Could you check a few things on this drawing? It's one solid part, dimensions in mm from its lowest x, y, z. A direction names the side the tool comes from. Give positions to 0.01 mm unless a question says otherwise; leave off trailing zeros. Order: outer loops, then holes, each group sorted by start corner. A loop starts at its lowest first (then second) coordinate and runs counter-clockwise, first axis right, second up. Notation, with made-up numbers: (73.5, 26) -> (79.5, 26) arc R15 ccw to (79.5, 46) -> close; hole circle Ø6 at (-31, -1). An arc over 180 degrees is marked (long way). Use one line per item in the form item = value. Start each with the question number.
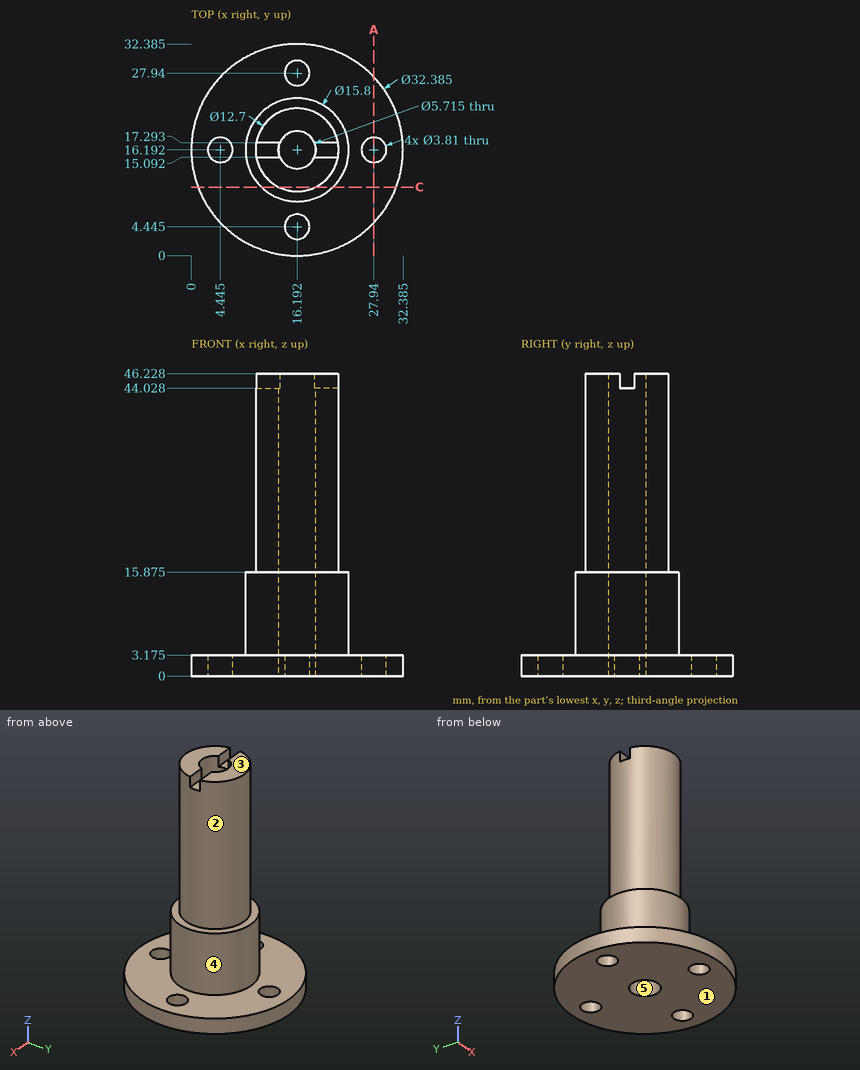
(1) Imagine slicing it at A-A (x = 27.94). Write out the boundary of the cut face in (y, z) (1 decimal).
(2) Please list where these lines run through material, in increasing order: probe 1 along Y at (x, z) = (16, 43.5) (1 decimal); probe 2 along Z at (x, y) = (18, 2) (1 decimal); probe 3 along X at (y, z) = (18, 25.5) (1 decimal).
(3) We'd pull the mould along X, two halves only. Please class the marked faces 3, 4 and 5: pulls with the +X half, pulls with the -X half, needs draft (parallel to the pull), parting line crosses it, or undercut.
(4) I'm going to push flat-ended pins straight in: pin 1 Ø6 at (y, z) = (7.5, 8) entering from -X (1 decimal); pin 2 Ø1.1 at (x, z) = (12, 45) entering from -Y; pin 3 Ø0.7 at (x, z) = (21.5, 44.5) entering from -Y (1 decimal). Where does each tip first touch, or does it pass through?
(5) Which directions (+Z, -Z, +X, -X, +Y, -Y) give clear straight access to the entire face, cutting with the end or side of a thin tool? Please do the marked faces 1 and 2.
(6) Imagine slicing it at C-C (y = 10.5). Write out the boundary of the cut face in (x, z) (1 decimal).
Calculated:
q1.outline = (5, 0) -> (14.3, 0) -> (14.3, 3.2) -> (5, 3.2) -> close; (18.1, 0) -> (27.3, 0) -> (27.3, 3.2) -> (18.1, 3.2) -> close
q2.probe_1 = 9.8 to 13.3, 19 to 22.5
q2.probe_2 = 0 to 3.2
q2.probe_3 = 10.1 to 14, 18.4 to 22.3
q3.face_3 = needs draft
q3.face_4 = parting line crosses it
q3.face_5 = undercut
q4.pin_1 = 10.7
q4.pin_2 = 10.99
q4.pin_3 = 12.2
q5.face_1 = -Z, +X, -X, +Y, -Y
q5.face_2 = +Z
q6.outline = (1, 0) -> (31.4, 0) -> (31.4, 3.2) -> (21.7, 3.2) -> (21.7, 15.9) -> (19, 15.9) -> (19, 46.2) -> (13.4, 46.2) -> (13.4, 15.9) -> (10.7, 15.9) -> (10.7, 3.2) -> (1, 3.2) -> close
